```python
from build123d import *


with BuildPart() as part:
    # Sketch 1 → Revolve 1 (revolve)
    with BuildSketch(Plane(origin=(0, 0, 0), x_dir=(1, 0, 0), z_dir=(0, 1, 0)), mode=Mode.PRIVATE) as revolve_1_sk:
        with BuildLine():
            Line((-21, -20), (0, -20))
            Line((0, -20), (0, 76.509456591))
            add(Edge.make_bspline(
                [(-21, 23.303526799), (-20.950151988, 23.55619715), (-20.588242456, 25.356689417), (-19.861805291, 28.542980585), (-18.781007648, 32.618309393), (-17.683803917, 36.387694686), (-16.794111183, 39.324775715), (-16.139995318, 41.546015667), (-15.635538449, 43.197589032), (-15.024163935, 45.012380328), (-13.937228163, 47.886209516), (-11.955046686, 52.531179902), (-8.996626021, 58.945239937), (-6.340494309, 64.415530495), (-4.283171781, 68.509695264), (-2.81904039, 71.351111958), (-1.479938004, 73.873249362), (-0.567336195, 75.524317414), (-0.112134261, 76.316693352), (0, 76.509456591)],
                knots=[0.246223276, 0.246223276, 0.246223276, 0.246223276, 0.255865129, 0.31540599, 0.374946852, 0.434487714, 0.494028576, 0.523799007, 0.553569438, 0.583339868, 0.613110299, 0.672651161, 0.732192023, 0.791732885, 0.821503316, 0.851273747, 0.881044177, 0.910814608, 0.921120543, 0.921120543, 0.921120543, 0.921120543], degree=3))
            Line((-21, 23.303526799), (-21, -20))
        make_face()
    revolve(revolve_1_sk.sketch.rotate(Axis((0, 0, -76.509456591), (0, 0, 1)), 180), axis=Axis((0, 0, -76.509456591), (0, 0, 1)))

    # Sketch 2 → Cut-Revolve 1 (revolve, cut)
    with BuildSketch(Plane(origin=(0, 0, 0), x_dir=(1, 0, 0), z_dir=(0, 1, 0))):
        Polygon((21, -20), (21, 66.971973821), (16.441991992, 66.971973821), align=None)
    revolve(axis=Axis((0, 0, 20), (0, 0, -1)), mode=Mode.SUBTRACT)

    # Sketch 3 → Cut-Revolve 2 (revolve, cut)
    with BuildSketch(Plane(origin=(0, 0, 0), x_dir=(1, 0, 0), z_dir=(0, 1, 0))):
        with BuildLine():
            Line((1e-08, 76.509474859), (1e-08, 74.388246536))
            ThreePointArc((1e-08, 74.388246536), (1.026734817, 74.10458439), (1.762223825, 73.334062167))
            Line((1.762223825, 73.334062167), (4.025925166, 73.334062167))
            Line((4.025925166, 73.334062167), (4.025925166, 76.509474859))
            Line((4.025925166, 76.509474859), (1e-08, 76.509474859))
        make_face()
    revolve(axis=Axis((1e-08, 0, -76.509474859), (0, 0, 1)), mode=Mode.SUBTRACT)


solid = part.part
```
Could you check a few things on this model? Use its own coordinates, in mm. Round coordinates to 2 decimals unless told otherwise and drop trailing zeros. Loops run counter-clockwise (first coordinate to the right, second up) from the corner with the lowest first, then second, coordinate; pieces in that order, holes last.
Q1. Please list where these lines run through material, in increasing order: L1, parallel to X at y = -10.5, z = -22.5; L2, parallel to Z at x = 7.5, y = 12.5; L3, parallel to X at y = -2.5, z = -49.
Q2. For P1, Ø12, axis at y = 6, z = -58.5, coming from the +X side; P2, Ø3, axis at x = -12, z = -17, coming from the +Y side; P3, Ø4, axis at x = 12.5, z = 4.5, coming from the +Y side, each with a flat end and sliding along its axis, tell me the tip position at first contact or that it passes through.
Q3. I want a section at A-A (z = 9). Write out the boundary of the cut face in (x, y), and give its area (3 significant figures).
Q4. I want a section at B-B (z = -6). Write out the boundary of the cut face in (x, y), and give its area (3 significant figures).
Answer below:
1. L1: x = -15.56 to 15.56
1. L2: z = -46.18 to 20
1. L3: x = -13.21 to 13.21
2. P1: stops at x = 11.18
2. P2: stops at y = 15.91
2. P3: stops at y = 17.25
3. outline: circle Ø40.85 at (0, 0)
3. area: 1,310 mm2
4. outline: circle Ø39.27 at (0, 0)
4. area: 1,210 mm2
